```python
from build123d import *

# Parameters (mm, degrees)
F1_DEPTH = 2.032
F3_DEPTH = 99.352875


with BuildPart() as f1:
    # F0 (on Top) → F1 (new body)
    with BuildSketch(Plane.XY):
        Polygon((49.6764375, -6.35), (49.6764375, 6.35), (-44.5964375, 6.35), (-49.6764375, -6.35), align=None)
    extrude(amount=F1_DEPTH)

    # F2 (on face) → F3 (join, through all)
    with BuildSketch(Plane.YZ.offset(49.6764375)):
        Polygon((-6.35, 0), (-6.35, 2.032), (-8.4541975976, 0), align=None)
    extrude(amount=-F3_DEPTH)


solid = f1.part
```
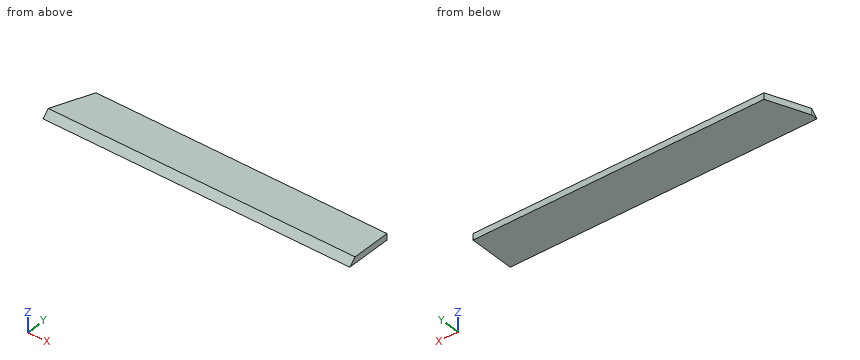
The listing builds one solid part. Answer for the finished solid, in the listing's coordinates (mm). Give positions to 0.01 mm unless a question says otherwise; leave off trailing zeros. Order: outer loops, then holes, each group sorted by start corner. A loop starts at its lowest first (then second) coordinate and runs counter-clockwise, first axis right, second up. Notation, with made-up numbers: (69, 46.25) -> (121, 46.25) arc R17 ccw to (121, 56.25) -> close; hole circle Ø1 at (-30, 60). An arc over 180 degrees is marked (long way). One line per item, written item: value.
1) Find section B-B, the plane x = -36. Determine the outline of the cut face in (y, z).
Reported:
outline: (-8.45, 0) -> (6.35, 0) -> (6.35, 2.03) -> (-6.35, 2.03) -> close
2) Find section A-A, the plane z = 0.65. Determine the outline of the cut face in (x, y).
Reported:
outline: (-49.68, -7.78) -> (49.68, -7.78) -> (49.68, 6.35) -> (-44.6, 6.35) -> (-49.68, -6.35) -> close
3) Find section C-C, the plane y = 0.5. Determine the outline of the cut face in (x, z).
Reported:
outline: (-46.94, 0) -> (49.68, 0) -> (49.68, 2.03) -> (-46.94, 2.03) -> close
4) A flat-ended cylindrical pin translates along its axis: P1, Ø1, axis at x = -17, z = 1.5, coming from the -Y side. Find the tip coordinate at first contact, or state that the pin passes through.
Reported:
P1: stops at y = -7.42
5) Find the intervals of material crossed by line 1 (X direction, y = -1.75, z = 0.9); line 2 (X direction, y = -1.5, z = 0.65); line 3 (Y direction, x = -6, z = 0.85), in increasing order.
Reported:
line 1: x = -47.84 to 49.68
line 2: x = -47.74 to 49.68
line 3: y = -7.57 to 6.35
